from build123d import *

# Parameters (mm, degrees)
EXTRUDE_1_DEPTH     = 2
SKETCH_3_R          = 1.55
CUT_EXTRUDE_1_DEPTH = 2


with BuildPart() as part:
    # Эскиз1 → Бобышка-Вытянуть1 (new body)
    with BuildSketch(Plane.XY):
        Polygon((0, 0), (-293.143158486, -169.261155122), (-111.86100446, -273.906060772), (0, -209.31740407), align=None)
    extrude(amount=EXTRUDE_1_DEPTH)

    # Эскиз3 → Вырез-Вытянуть1 (cut)
    with BuildSketch(Plane(origin=(0, 0, 0), x_dir=(-1, 0, 0), z_dir=(0, 0, -1))):
        with Locations((12.682716025, -25.001847817)):
            Circle(SKETCH_3_R)
        with Locations((12.682716025, -198.961582281)):
            Circle(SKETCH_3_R)
        with Locations((114.489281174, -257.744795592)):
            Circle(SKETCH_3_R)
        with Locations((265.149449722, -170.776394274)):
            Circle(SKETCH_3_R)
    extrude(amount=-CUT_EXTRUDE_1_DEPTH, mode=Mode.SUBTRACT)


solid = part.part
CAD build for the part. Positions are in the model's coordinates, mm. Give positions to 0.01 mm unless a question says otherwise; leave off trailing zeros. Loops run counter-clockwise (first coordinate to the right, second up) from the corner with the lowest first, then second, coordinate; pieces in that order, holes last. Notation, with made-up numbers: M -12,21.25 L 27,21.25 A20 ccw 27,51.25 Z; hole C 87,47 d7. An arc over 180 degrees is marked long. Write each question's results on one line, items separated by ' | '.
Q1. Band-saw the part on C-C on y = -37. Write the cut outline in (x, z).
Geometry check:
outline: M -64.08,0 L 0,0 L 0,2 L -64.08,2 Z
Q2. Probe probe 1 along Y at (x, z) = (-160.5, 1.8); probe 2 along Y at (x, z) = (-96.5, 1.5); probe 3 along X at (y, z) = (-244.5, 0.7). List the from-to ranges inside material, lowest first.
Geometry check:
probe 1: y = -245.83 to -92.67 | probe 2: y = -265.04 to -55.72 | probe 3: x = -162.8 to -60.93
Q3. Band-saw the part on A-A on z = 1.65. Write the cut outline in (x, y).
Geometry check:
outline: M -293.14,-169.26 L -111.86,-273.91 L 0,-209.32 L 0,0 Z; hole C -265.15,-170.78 d3.1; hole C -114.49,-257.74 d3.1; hole C -12.68,-198.96 d3.1; hole C -12.68,-25 d3.1
Q4. Flat gauge pins, fed straight in: P1, Ø1.9, axis at x = -12.68, y = -198.96, coming from the -Z side; P2, Ø1, axis at y = -239, z = 1.5, coming from the -X side. Where does each tip first touch, or does it go through?
Geometry check:
P1: passes through | P2: stops at x = -173.2
Q5. Band-saw the part on B-B on x = -39. Write the cut outline in (y, z), and give its area (3 significant figures).
Geometry check:
outline: M -231.84,0 L -22.52,0 L -22.52,2 L -231.84,2 Z | area: 419 mm²
